Part model, mm, in its own coordinate system. A direction names the side the tool comes from. Coordinates: 2 decimals unless noted, no trailing zeros. Loops run counter-clockwise (first coordinate to the right, second up) from the corner with the lowest first, then second, coordinate; pieces in that order, holes last. Notation, with made-up numbers: (69, 64) - (118, 64) arc R12 ccw to (118, 79) - close; hole circle Ø8 at (68, 66.5). An arc over 180 degrees is marked (long way). One line per question, with ' | ' between items. Start each with the question number.
from build123d import *

# Parameters (mm, degrees)
SKETCH1_W            = 50
SKETCH1_H            = 35
SKETCH1_R            = 9.5
SKETCH1_R_2          = 1.5
BOSS_EXTRUDE3_DEPTH  = 6
SKETCH4_W            = 50
SKETCH4_H            = 35
BOSS_EXTRUDE5_DEPTH  = 2
BOSS_EXTRUDE6_DEPTH  = 55
BOSS_EXTRUDE9_DEPTH  = 69
BOSS_EXTRUDE10_DEPTH = 8
SKETCH9_R            = 2
CUT_EXTRUDE1_DEPTH   = 8.5


with BuildPart() as part:
    # Sketch1 → Boss-Extrude3 (new body)
    with BuildSketch(Plane.XY):
        with Locations((25, 17.5)):
            Rectangle(SKETCH1_W, SKETCH1_H)
        with Locations((32.5, 17.5)):
            Circle(SKETCH1_R, mode=Mode.SUBTRACT)
        with Locations((41.692388155, 26.692388155)):
            Circle(SKETCH1_R_2, mode=Mode.SUBTRACT)
        with Locations((41.692388155, 8.307611845)):
            Circle(SKETCH1_R_2, mode=Mode.SUBTRACT)
        with Locations((23.307611845, 8.307611845)):
            Circle(SKETCH1_R_2, mode=Mode.SUBTRACT)
        with Locations((23.307611845, 26.692388155)):
            Circle(SKETCH1_R_2, mode=Mode.SUBTRACT)
    extrude(amount=BOSS_EXTRUDE3_DEPTH)

    # Sketch4 → Boss-Extrude5 (add)
    with BuildSketch(Plane.XY.offset(6)):
        with Locations((25, 17.5)):
            Rectangle(SKETCH4_W, SKETCH4_H)
        with BuildLine():
            ThreePointArc((26.299419693, 26.47083501), (21.186291501, 28.813708499), (23.52916499, 23.700580307))
            ThreePointArc((23.52916499, 23.700580307), (23.763454109, 23.57743344), (23.755822455, 23.312861521))
            ThreePointArc((23.755822455, 23.312861521), (22, 17.5), (23.755822455, 11.687138479))
            ThreePointArc((23.755822455, 11.687138479), (23.763454109, 11.42256656), (23.52916499, 11.299419693))
            ThreePointArc((23.52916499, 11.299419693), (21.186291501, 6.186291501), (26.299419693, 8.52916499))
            ThreePointArc((26.299419693, 8.52916499), (26.42256656, 8.763454109), (26.687138479, 8.755822455))
            ThreePointArc((26.687138479, 8.755822455), (32.5, 7), (38.312861521, 8.755822455))
            ThreePointArc((38.312861521, 8.755822455), (38.57743344, 8.763454109), (38.700580307, 8.52916499))
            ThreePointArc((38.700580307, 8.52916499), (43.813708499, 6.186291501), (41.47083501, 11.299419693))
            ThreePointArc((41.47083501, 11.299419693), (41.236545891, 11.42256656), (41.244177545, 11.687138479))
            ThreePointArc((41.244177545, 11.687138479), (43, 17.5), (41.244177545, 23.312861521))
            ThreePointArc((41.244177545, 23.312861521), (41.236545891, 23.57743344), (41.47083501, 23.700580307))
            ThreePointArc((41.47083501, 23.700580307), (43.813708499, 28.813708499), (38.700580307, 26.47083501))
            ThreePointArc((38.700580307, 26.47083501), (38.57743344, 26.236545891), (38.312861521, 26.244177545))
            ThreePointArc((38.312861521, 26.244177545), (32.5, 28), (26.687138479, 26.244177545))
            ThreePointArc((26.687138479, 26.244177545), (26.42256656, 26.236545891), (26.299419693, 26.47083501))
        make_face(mode=Mode.SUBTRACT)
    extrude(amount=BOSS_EXTRUDE5_DEPTH)

    # Sketch8 → Boss-Extrude6 (add)
    with BuildSketch(Plane(origin=(0, 0, 0), x_dir=(-1, 0, 0), z_dir=(0, 0, -1))):
        with BuildLine():
            Line((-8.5, 35), (-22.740329685, 35))
            Line((-22.740329685, 35), (-22.740329685, 30.367452558))
            ThreePointArc((-22.740329685, 30.367452558), (-20.171344576, 27.9320063), (-18.194683381, 24.99535966))
            Line((-18.194683381, 24.99535966), (-18.194683381, 25))
            Line((-18.194683381, 25), (-8.5, 25))
            Line((-8.5, 25), (-8.5, 10.000000197))
            Line((-8.5, 10.000000197), (-18.197115572, 10.000000197))
            ThreePointArc((-18.197115572, 10.000000197), (-20.17303677, 7.065994176), (-22.740329685, 4.632547442))
            Line((-22.740329685, 4.632547442), (-22.740329685, 0))
            Line((-22.740329685, 0), (-8.5, 0))
            Line((-8.5, 0), (0, 0))
            Line((0, 0), (0, 10.000000197))
            Line((0, 10.000000197), (0, 25))
            Line((0, 25), (0, 35))
            Line((0, 35), (-8.5, 35))
        make_face()
    extrude(amount=BOSS_EXTRUDE6_DEPTH)

    # Sketch13 → Boss-Extrude9 (add)
    with BuildSketch(Plane(origin=(0, 0, -55), x_dir=(-1, 0, 0), z_dir=(0, 0, -1))):
        with BuildLine():
            Line((-8.5, 25), (-8.5, 10))
            Line((-8.5, 10), (-19.509618943, 10))
            ThreePointArc((-19.509618943, 10), (-20.959823947, 7.917498413), (-22.740329685, 6.109265373))
            Line((-22.740329685, 6.109265373), (-22.740329685, 0))
            Line((-22.740329685, 0), (0, 0))
            Line((0, 0), (0, 35))
            Line((0, 35), (-22.740329685, 35))
            Line((-22.740329685, 35), (-22.740329685, 28.890734627))
            ThreePointArc((-22.740329685, 28.890734627), (-20.959823947, 27.082501587), (-19.509618943, 25))
            Line((-19.509618943, 25), (-8.5, 25))
        make_face()
    extrude(amount=BOSS_EXTRUDE9_DEPTH)

    # Sketch14 → Boss-Extrude10 (add)
    with BuildSketch(Plane(origin=(0, 0, -124), x_dir=(-1, 0, 0), z_dir=(0, 0, -1))):
        with BuildLine():
            Line((-24.5, 17.5), (-24.5, 35))
            Line((-24.5, 35), (0, 35))
            Line((0, 35), (0, 0))
            Line((0, 0), (-50, 0))
            Line((-50, 0), (-50, 17.5))
            Line((-50, 17.5), (-40.5, 17.5))
            ThreePointArc((-40.5, 17.5), (-32.5, 9.5), (-24.5, 17.5))
        make_face()
    extrude(amount=BOSS_EXTRUDE10_DEPTH)

    # Sketch9 → Cut-Extrude1 (cut)
    with BuildSketch(Plane.ZY):
        with Locations((-7, 17.5)):
            Circle(SKETCH9_R)
        with Locations((-24, 17.5)):
            Circle(SKETCH9_R)
        with Locations((-41, 17.5)):
            Circle(SKETCH9_R)
        with Locations((-58, 17.5)):
            Circle(SKETCH9_R)
        with Locations((-75, 17.5)):
            Circle(SKETCH9_R)
        with Locations((-92, 17.5)):
            Circle(SKETCH9_R)
        with Locations((-109, 17.5)):
            Circle(SKETCH9_R)
    extrude(amount=-CUT_EXTRUDE1_DEPTH, mode=Mode.SUBTRACT)


solid = part.part
1) Wall check: line 1 along Y through (x, z) = (15, -52); line 2 along Z through (x, y) = (23, 1); line 3 along Y through (x, z) = (3, -92). Give the ranges that are in metal, low to high. Write a range as [from, to].
2) Tool access for faces 4 (the cylindrical face through (20.983, 27.11, -89.017)), 5 (the flat face through (19, 14, -132)), 6 (the cylindrical face through (21.115, 6.26, 6.986)): list every direction of +Z, -Z, +X, -X, +Y, -Y with a clear straight run to the whole face (end or side of a thin tool).
3) Band-saw the part on C-C on z = -121.5. List the corners of the cut face in (x, y), then the cut area to 3 significant figures.
4) Mould opens along Y. For faces 1 (the flat face through (50, 9, -128)), 2 (the flat face through (20.6, 27.5, -55)), 3 (the flat face through (40, 11, 6)) say: +Y half, -Y half, draft (parallel to the pull), parting line (faces both ways), or undercut.
5) Band-saw the part on B-B on x = 32.5. List the corners of the cut face in (y, z), then the cut area to 3 significant figures.
6) Pin check, flat tips, straight feed: pin 1 Ø3 at (y, z) = (17.5, -58) entering from -X; pin 2 Ø9 at (x, z) = (44, -126.5) entering from +Y; pin 3 Ø3 at (y, z) = (31, -71.5) entering from +X; pin 4 Ø2.5 at (y, z) = (23.5, -129.5) entering from +X. Stop position of each tip, or through.
7) Band-saw the part on D-D on z = -92. List the corners of the cut face in (x, y).
Values found:
1) line 1: [0, 10], [25, 35] | line 2: [-132, -124], [0, 8] | line 3: [0, 15.5], [19.5, 35]
2) face 4: +X | face 5: -Z, +X, -X, +Y, -Y | face 6: +Z
3) outline: (0, 0) - (22.74, 0) - (22.74, 6.11) arc R15 cw to (19.51, 10) - (8.5, 10) - (8.5, 25) - (19.51, 25) arc R15 cw to (22.74, 28.89) - (22.74, 35) - (0, 35) - close | area: 568 mm²
4) face 1: draft | face 2: undercut | face 3: undercut
5) outline: (0, -132) - (9.5, -132) - (9.5, -124) - (0, -124) - close; (0, 0) - (8, 0) - (8, 6) - (7, 6) - (7, 8) - (0, 8) - close; (27, 0) - (35, 0) - (35, 8) - (28, 8) - (28, 6) - (27, 6) - close | area: 200 mm²
6) pin 1: through | pin 2: y = 17.5 | pin 3: x = 22.74 | pin 4: x = 24.5
7) outline: (0, 0) - (22.74, 0) - (22.74, 6.11) arc R15 cw to (19.51, 10) - (8.5, 10) - (8.5, 15.5) - (0, 15.5) - close; (0, 19.5) - (8.5, 19.5) - (8.5, 25) - (19.51, 25) arc R15 cw to (22.74, 28.89) - (22.74, 35) - (0, 35) - close
